Work out the finished part from the listing and answer in its coordinate system (mm). A direction names the side the tool comes from. Coordinates: 2 decimals unless noted, no trailing zeros. Write each loop counter-clockwise with the first axis right and the second up, starting at its lowest first coordinate (ties: lowest second). Pieces come first, ordered by that corner, then holes. Notation, with made-up numbers: (-7, 81.25) - (25, 81.25) arc R12 ccw to (25, 89.25) - close; hole circle Ø5 at (76.25, 31.25). An arc over 180 degrees is marked (long way). One line per item, written item: value.
```python
from build123d import *

# Parameters (mm, degrees)
F1_DEPTH  = 5.5
F3_DEPTH  = 7
F5_DEPTH  = 5.5
F6_R      = 10
F7_DEPTH  = 5.5
F8_R      = 10
F9_DEPTH  = 5.5
F11_DEPTH = 12.501
F12_R     = 1.5
F13_DEPTH = 18.001
F14_R     = 2.5
F15_DEPTH = 1.5
F16_R     = 2.5
F17_DEPTH = 1.5
F18_R     = 83.4133197042
F19_DEPTH = 12.5


with BuildPart() as f1:
    # F0 (on Right) → F1 (new body)
    with BuildSketch(Plane.YZ):
        with BuildLine():
            ThreePointArc((42.0884551059, 9.566760493), (22.2278404433, 6.393975856), (2.2496848399, 8.7142938969))
            ThreePointArc((2.2496848399, 8.7142938969), (-9, 0), (2.2496848399, -8.7142938969))
            ThreePointArc((2.2496848399, -8.7142938969), (22.2278404433, -6.393975856), (42.0884551059, -9.566760493))
            ThreePointArc((42.0884551059, -9.566760493), (55, 0), (42.0884551059, 9.566760493))
        make_face()
    extrude(amount=F1_DEPTH)

    # F2 (on face) → F3 (join)
    with BuildSketch(Plane.YZ.offset(5.5)):
        with BuildLine():
            ThreePointArc((42.0884551059, 9.566760493), (22.2278404433, 6.393975856), (2.2496848399, 8.7142938969))
            ThreePointArc((2.2496848399, 8.7142938969), (1.1338771821, 8.9282877718), (0, 9))
            Line((0, 9), (0, 7))
            ThreePointArc((0, 7), (3.4468203516, 6.0925716626), (6, 3.6055512755))
            Line((6, 3.6055512755), (12.2854984686, -6.8541504262))
            ThreePointArc((12.2854984686, -6.8541504262), (27.3262576199, -6.6802021184), (42.0884551059, -9.566760493))
            ThreePointArc((42.0884551059, -9.566760493), (55, 0), (42.0884551059, 9.566760493))
        make_face()
    extrude(amount=F3_DEPTH)

    # F4 (on face) → F5 (join)
    with BuildSketch(Plane.YZ.offset(12.5)):
        with BuildLine():
            ThreePointArc((2.2496848399, 8.7142938969), (1.1338771821, 8.9282877718), (0, 9))
            ThreePointArc((0, 9), (-8.9282877718, -1.1338771821), (2.2496848399, -8.7142938969))
            ThreePointArc((2.2496848399, -8.7142938969), (7.235317588, -7.610097682), (12.2854984686, -6.8541504262))
            ThreePointArc((12.2854984686, -6.8541504262), (27.3262576199, -6.6802021184), (42.0884551059, -9.566760493))
            ThreePointArc((42.0884551059, -9.566760493), (55, 0), (42.0884551059, 9.566760493))
            ThreePointArc((42.0884551059, 9.566760493), (22.2278404433, 6.393975856), (2.2496848399, 8.7142938969))
        make_face()
    extrude(amount=F5_DEPTH)

    # F6 (on face) → F7 (cut)
    with BuildSketch(Plane.YZ.offset(18)):
        with Locations((45, 0)):
            Circle(F6_R)
    extrude(amount=-F7_DEPTH, mode=Mode.SUBTRACT)

    # F8 (on face) → F9 (cut)
    with BuildSketch(Plane(origin=(0, 0, 0), x_dir=(0, -1, 0), z_dir=(-1, 0, 0))):
        with Locations((-45, 0)):
            Circle(F8_R)
    extrude(amount=-F9_DEPTH, mode=Mode.SUBTRACT)

    # F10 (on face) → F11 (cut, through all)
    with BuildSketch(Plane.YZ.offset(12.5)):
        with BuildLine():
            ThreePointArc((45, 8), (52.7274066103, 2.0705523608), (49, -6.9282032303))
            Line((49, -6.9282032303), (43.8038475773, -9.9282032303))
            ThreePointArc((43.8038475773, -9.9282032303), (54.9820346699, -0.5991526088), (45, 10))
            Line((45, 10), (45, 8))
        make_face()
    extrude(amount=-F11_DEPTH, mode=Mode.SUBTRACT)

    # F12 (on face) → F13 (cut, through all)
    with BuildSketch(Plane.YZ.offset(18)):
        Circle(F12_R)
        with Locations((45, 0)):
            Circle(F12_R)
    extrude(amount=-F13_DEPTH, mode=Mode.SUBTRACT)

    # F14 (on face) → F15 (cut)
    with BuildSketch(Plane.YZ.offset(18)):
        Circle(F14_R)
    extrude(amount=-F15_DEPTH, mode=Mode.SUBTRACT)

    # F16 (on face) → F17 (cut)
    with BuildSketch(Plane(origin=(0, 0, 0), x_dir=(0, -1, 0), z_dir=(-1, 0, 0))):
        Circle(F16_R)
    extrude(amount=-F17_DEPTH, mode=Mode.SUBTRACT)

    # F18 (on Top) → F19 (cut, symmetric)
    with BuildSketch(Plane.XY):
        with Locations((-81, 22.1690699729)):
            Circle(F18_R)
        with Locations((99, 22.1690699729)):
            Circle(F18_R)
    extrude(amount=F19_DEPTH, both=True, mode=Mode.SUBTRACT)


solid = f1.part
```
Item 1: Which of the six approach directions +Z, -Z, +X, -X, +Y, -Y give full straight-line access (tool end or side, diameter ignored) to faces 1 (the face through (9, 0, 8)), 2 (the face through (0.74, 0.54, -2.44)), 3 (the face through (17.26, -0.54, -2.44)), 4 (the face through (12.5, 42, 0))?
Evaluation:
face 1: +Z, -Z, -Y
face 2: -X
face 3: +X
face 4: +X, +Y
Item 2: Given pin 1 (6 mm diameter, centred on y = 0, z = 0, fed in from +X); pin 2 (5 mm diameter, centred on y = 45, z = 0, fed in from -X); pin 3 (6 mm diameter, centred on x = 11.5, z = -4.5, fed in from -Y); pin 4 (4 mm diameter, centred on y = 0, z = 0, fed in from -X), each flat-ended and moving along its own axis, determine where each tip first touches the part or whether it passes through.
Evaluation:
pin 1: stops at x = 18
pin 2: stops at x = 5.5
pin 3: stops at y = -8.84
pin 4: stops at x = 1.5
Item 3: Section D-D, the plane z = 0 is taken. Give the number of separate pieces and of enclosed holes in the cut face, then the cut area to 3 significant figures.
Evaluation:
separate pieces: 4
enclosed holes: 0
area: 620 mm2
Item 4: Section C-C, the plane y = 8.5 is taken. Determine the outline of the cut face in (x, z), then the cut area to 3 significant figures.
Evaluation:
outline: (1.29, -7.39) - (5.5, -7.39) - (5.5, -0.55) - (12.5, -0.55) - (12.5, -7.39) - (16.71, -7.39) - (16.71, 7.39) - (1.29, 7.39) - close
area: 180 mm2
Item 5: Section B-B, the plane x = 7.25 is taken. Determine the outline of the cut face in (y, z), then the cut area to 3 significant figures.
Evaluation:
outline: (0, 7) arc R7 cw to (6, 3.61) - (12.29, -6.85) arc R73.62 cw to (42.09, -9.57) arc R10 ccw to (43.8, -9.93) - (49, -6.93) arc R8 ccw to (45, 8) - (45, 10) arc R10 ccw to (42.09, 9.57) arc R73.62 cw to (2.25, 8.71) arc R9 ccw to (0, 9) - close; hole circle Ø3 at (45, 0)
area: 651 mm2
Item 6: Section A-A, the plane z = -8 is taken. Determine the outline of the cut face in (x, y), then the cut area to 3 significant figures.
Evaluation:
outline: (0, -4.12) - (5.5, -4.12) - (5.5, 5.28) - (0.69, 5.28) arc R83.41 cw to (0, 2.25) - close; (0.7, 39) arc R83.41 cw to (1.25, 36.03) - (16.75, 36.03) arc R83.41 cw to (17.3, 39) - (12.5, 39) - (12.5, 47.14) - (5.5, 47.14) - (5.5, 39) - close; (12.5, -4.12) - (18, -4.12) - (18, 2.25) arc R83.41 cw to (17.31, 5.28) - (12.5, 5.28) - close
area: 206 mm2
Item 7: Determine the mould class of faces 5 (the face through (16.5, 0, -2)), 6 (the face through (18, -3, 0)), 7 (the face through (8.951, 43.549, 9.894)), 8 (the face through (2.28, 17.42, -0.13)) for opening direction Y: +Y half, -Y half, draft (parallel to the pull), parting line (faces both ways), or undercut.
Evaluation:
face 5: undercut
face 6: draft
face 7: -Y half
face 8: undercut
Item 8: Consider probe 1 along X at (y, z) = (-6, 1.75); probe 2 along Z at (x, y) = (1.1, 0); probe 3 along X at (y, z) = (19.5, 2.5). Determine where each line is inside the solid, lowest interval first.
Evaluation:
probe 1: x = 0 to 5.5, 12.5 to 18
probe 2: z = -9 to -2.5, 2.5 to 9
probe 3: x = 2.37 to 15.63
